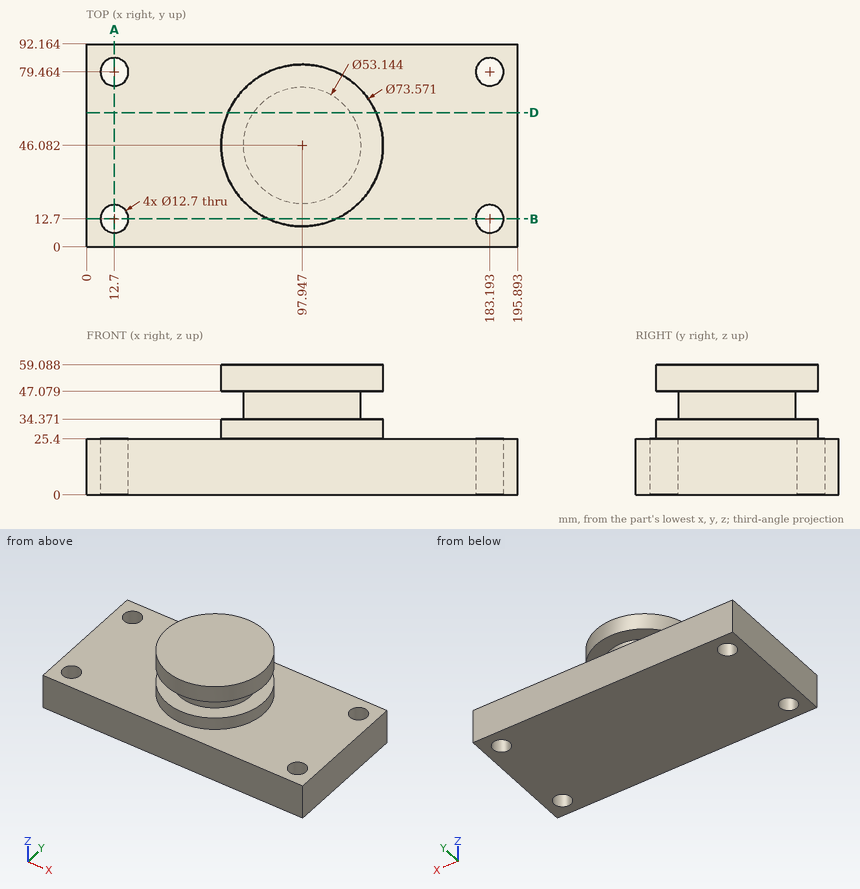
Check sheet for the drawn part. Datum: minimum x, y, z corner. Units: mm. Give positions to 0.01 mm unless a question says otherwise; leave off trailing zeros. Order: outer loops, then holes, each group sorted by start corner. A loop starts at its lowest first (then second) coordinate and runs counter-clockwise, first axis right, second up. Notation, with made-up numbers: (63.5, 54) -> (108.5, 54) arc R8 cw to (108.5, 64) -> close; hole circle Ø9 at (57, 55.5). An arc over 180 degrees is marked (long way). Answer as CSV lines item,"result".
Q1. Sectioned sample at A-A on x = 12.7. Record the cut outline in (y, z), plus the area to 3 significant figures.
Solutions:
outline,"(0, 0) -> (6.35, 0) -> (6.35, 25.4) -> (0, 25.4) -> close; (19.05, 0) -> (73.11, 0) -> (73.11, 25.4) -> (19.05, 25.4) -> close; (85.81, 0) -> (92.16, 0) -> (92.16, 25.4) -> (85.81, 25.4) -> close"
area,"1,700 mm²"
Q2. Sectioned sample at B-B on y = 12.7. Record the cut outline in (x, z), plus the area to 3 significant figures.
Solutions:
outline,"(0, 0) -> (6.35, 0) -> (6.35, 25.4) -> (0, 25.4) -> close; (19.05, 0) -> (176.84, 0) -> (176.84, 25.4) -> (113.4, 25.4) -> (113.4, 34.37) -> (82.49, 34.37) -> (82.49, 25.4) -> (19.05, 25.4) -> close; (82.49, 47.08) -> (113.4, 47.08) -> (113.4, 59.09) -> (82.49, 59.09) -> close; (189.54, 0) -> (195.89, 0) -> (195.89, 25.4) -> (189.54, 25.4) -> close"
area,"4,980 mm²"
Q3. Scan lines: probe 1 along Y at (x, z) = (12.7, 10.75); probe 2 along Z at (x, y) = (97, 79.5); probe 3 along Z at (x, y) = (117.5, 86). Record each from-to range of solid material in increasing order.
Solutions:
probe 1,"y = 0 to 6.35, 19.05 to 73.11, 85.81 to 92.16"
probe 2,"z = 0 to 34.37, 47.08 to 59.09"
probe 3,"z = 0 to 25.4"
Q4. Depth check by flat-ended pin: pin 1 (14.5 mm diameter, centred on x = 12.7, y = 79.46, fed in from +Z); pin 2 (3 mm diameter, centred on y = 56, z = 39, fed in from +X); pin 3 (4 mm diameter, centred on y = 31, z = 38, fed in from -X); pin 4 (11.5 mm diameter, centred on x = 12.7, y = 12.7, fed in from +Z). Enter the tip coordinate at first touch or a pass-through.
Solutions:
pin 1,"stops at z = 25.4"
pin 2,"stops at x = 123.15"
pin 3,"stops at x = 74.82"
pin 4,"passes through"
Q5. Sectioned sample at D-D on y = 61. Record the cut outline in (x, z).
Solutions:
outline,"(0, 0) -> (195.89, 0) -> (195.89, 25.4) -> (131.57, 25.4) -> (131.57, 34.37) -> (119.94, 34.37) -> (119.94, 47.08) -> (131.57, 47.08) -> (131.57, 59.09) -> (64.32, 59.09) -> (64.32, 47.08) -> (75.96, 47.08) -> (75.96, 34.37) -> (64.32, 34.37) -> (64.32, 25.4) -> (0, 25.4) -> close"
